Can you work these out from the model? Positions are in its coordinate system, mm. A direction names the side the tool comes from. Give positions to 0.01 mm unless a question says otherwise; leave off trailing zeros. Order: outer loops, then holes, each group sorted by start corner. A loop starts at its lowest first (then second) coordinate and runs counter-clockwise, first axis right, second up. Notation, with made-up numbers: M 6,52.25 L 46,52.25 A22 cw 46,61.25 Z; hole C 2.5,37 d10. An arc over 180 degrees is marked long. Answer as a JSON object with one key per item and string values.
```python
from build123d import *

# Parameters (mm, degrees)
SKETCH2_R           = 21
BOSS_EXTRUDE1_DEPTH = 3.5
SKETCH4_R           = 5.5
SKETCH4_R_2         = 1.143
SKETCH4_R_3         = 1.5875
CUT_EXTRUDE2_DEPTH  = 4.5
SKETCH5_R           = 2.9
CUT_EXTRUDE4_DEPTH  = 2
SKETCH6_W           = 2.148549125
SKETCH6_H           = 1
SKETCH8_R           = 3.6
SKETCH8_W           = 3.4
SKETCH8_H           = 3.4
BOSS_EXTRUDE3_DEPTH = 15
SKETCH7_R           = 6.25
BOSS_EXTRUDE4_DEPTH = 2.5


with BuildPart() as part:
    # Sketch2 → Boss-Extrude1 (new body)
    with BuildSketch(Plane(origin=(0, 0, 0), x_dir=(1, 0, 0), z_dir=(0, 1, 0))):
        Circle(SKETCH2_R)
    extrude(amount=BOSS_EXTRUDE1_DEPTH)

    # Sketch4 → Cut-Extrude2 (cut, through all)
    with BuildSketch(Plane(origin=(0, 3.5, 0), x_dir=(1, 0, 0), z_dir=(0, 1, 0))):
        Circle(SKETCH4_R)
        with Locations((7.445, 0)):
            Circle(SKETCH4_R_2)
        with Locations((10.54, 0)):
            Circle(SKETCH4_R_2)
        with Locations((13.46, 0)):
            Circle(SKETCH4_R_2)
        with Locations((16.51, 0)):
            Circle(SKETCH4_R_2)
        with Locations((10, 10)):
            Circle(SKETCH4_R_3)
        with Locations((0, -7.445)):
            Circle(SKETCH4_R_2)
        with Locations((0, -10.54)):
            Circle(SKETCH4_R_2)
        with Locations((0, -13.46)):
            Circle(SKETCH4_R_2)
        with Locations((0, -16.51)):
            Circle(SKETCH4_R_2)
        with Locations((10, -10)):
            Circle(SKETCH4_R_3)
        with Locations((-7.445, 0)):
            Circle(SKETCH4_R_2)
        with Locations((-10.54, 0)):
            Circle(SKETCH4_R_2)
        with Locations((-13.46, 0)):
            Circle(SKETCH4_R_2)
        with Locations((-16.51, 0)):
            Circle(SKETCH4_R_2)
        with Locations((-10, -10)):
            Circle(SKETCH4_R_3)
        with Locations((0, 7.445)):
            Circle(SKETCH4_R_2)
        with Locations((0, 10.54)):
            Circle(SKETCH4_R_2)
        with Locations((0, 13.46)):
            Circle(SKETCH4_R_2)
        with Locations((0, 16.51)):
            Circle(SKETCH4_R_2)
        with Locations((-10, 10)):
            Circle(SKETCH4_R_3)
    extrude(amount=-CUT_EXTRUDE2_DEPTH, mode=Mode.SUBTRACT)

    # Sketch5 → Cut-Extrude4 (cut)
    with BuildSketch(Plane(origin=(0, 3.5, 0), x_dir=(1, 0, 0), z_dir=(0, 1, 0))):
        with Locations((-10, 10)):
            Circle(SKETCH5_R)
        with Locations((-10, -10)):
            Circle(SKETCH5_R)
        with Locations((10, 10)):
            Circle(SKETCH5_R)
        with Locations((10, -10)):
            Circle(SKETCH5_R)
    extrude(amount=-CUT_EXTRUDE4_DEPTH, mode=Mode.SUBTRACT)

    # Sketch6 → Revolve1 (revolve)
    with BuildSketch(Plane.XY):
        with Locations((-21.425725437, 3)):
            Rectangle(SKETCH6_W, SKETCH6_H)
    revolve(axis=Axis((0, 0, 0), (0, 1, 0)))



with BuildPart() as body_2:
    # Sketch8 → Boss-Extrude3 (new body)
    with BuildSketch(Plane(origin=(0, 0, 0), x_dir=(1, 0, 0), z_dir=(0, 1, 0))):
        Circle(SKETCH8_R)
        Rectangle(SKETCH8_W, SKETCH8_H, mode=Mode.SUBTRACT)
    extrude(amount=BOSS_EXTRUDE3_DEPTH)


with BuildPart() as part_1:
    add(part.part)

    add(body_2.part)  # Boss-Extrude4 merges body 2
    # Sketch7 → Boss-Extrude4 (add)
    with BuildSketch(Plane(origin=(0, 3.5, 0), x_dir=(1, 0, 0), z_dir=(0, 1, 0))):
        Circle(SKETCH7_R)
    extrude(amount=-BOSS_EXTRUDE4_DEPTH)


solid = part_1.part
```
1) I need wall thicknesses on L1, parallel to X at y = 7.5, z = 0; L2, parallel to Y at x = -7.5, z = -19.5; L3, parallel to X at y = 0.55, z = 10. Which ranges of each line are inside material? Lowest first, please.
Results found:
{"L1": "x = -3.6 to -1.7, 1.7 to 3.6", "L2": "y = 0 to 3.5", "L3": "x = -18.47 to -11.59, -8.41 to -1.01, 1.01 to 8.41, 11.59 to 18.47"}
2) Thinking about a two-plate mould opening in Z: for faces 4 (the face through (3.434, 9.17, -1.081)), 5 (the face through (11.596, 1.774, 0.438)), which applies, pulls with the +Z half, pulls with the -Z half, needs draft (parallel to the pull), parting line crosses it, or undercut?
Results found:
{"face 4": "parting line crosses it", "face 5": "undercut"}
3) I want a section at C-C on x = 17. Write out the boundary of the cut face in (y, z).
Results found:
{"outline": "M 0,-12.33 L 2.5,-12.33 L 2.5,-14.74 L 3.5,-14.74 L 3.5,-1.03 L 0,-1.03 Z; M 0,1.03 L 3.5,1.03 L 3.5,14.74 L 2.5,14.74 L 2.5,12.33 L 0,12.33 Z"}
4) For faces 1 (the face through (11.25, 1.5, 11.25)), 2 (the face through (0, 0.5, 1.7)), 3 (the face through (-10.207, 0.76, 8.426)), which set-ups out of +Z, -Z, +X, -X, +Y, -Y let a thin tool reach every point of the face, with its end or its side?
Results found:
{"face 1": "+Y", "face 2": "-Y", "face 3": "+Y, -Y"}
5) I want a section at B-B on z = -10.54. Write out the boundary of the cut face in (x, y), and give its area (3 significant figures).
Results found:
{"outline": "M -19.88,2.5 L -18.16,2.5 L -18.16,0 L -11.49,0 L -11.49,1.5 L -12.85,1.5 L -12.85,3.5 L -19.88,3.5 Z; M -8.51,0 L -1.14,0 L -1.14,3.5 L -7.15,3.5 L -7.15,1.5 L -8.51,1.5 Z; M 1.14,0 L 8.51,0 L 8.51,1.5 L 7.15,1.5 L 7.15,3.5 L 1.14,3.5 Z; M 11.49,0 L 18.16,0 L 18.16,2.5 L 19.88,2.5 L 19.88,3.5 L 12.85,3.5 L 12.85,1.5 L 11.49,1.5 Z", "area": "90.8 mm²"}
6) I want a section at D-D on x = -10.54. Write out the boundary of the cut face in (y, z).
Results found:
{"outline": "M 0,-18.16 L 2.5,-18.16 L 2.5,-19.88 L 3.5,-19.88 L 3.5,-12.85 L 1.5,-12.85 L 1.5,-11.49 L 0,-11.49 Z; M 0,-8.51 L 1.5,-8.51 L 1.5,-7.15 L 3.5,-7.15 L 3.5,-1.14 L 0,-1.14 Z; M 0,1.14 L 3.5,1.14 L 3.5,7.15 L 1.5,7.15 L 1.5,8.51 L 0,8.51 Z; M 0,11.49 L 1.5,11.49 L 1.5,12.85 L 3.5,12.85 L 3.5,19.88 L 2.5,19.88 L 2.5,18.16 L 0,18.16 Z"}
7) I'm going to push flat-ended pins straight in: pin 1 Ø2 at (x, z) = (0, -7.445) entering from -Y; pin 2 Ø3.5 at (x, z) = (-10, 10) entering from +Y; pin 3 Ø6.5 at (x, z) = (11, 10.5) entering from +Y; pin 4 Ø1 at (x, y) = (0, 9) entering from +Z. Where does each tip first touch, or does it pass through?
Results found:
{"pin 1": "passes through", "pin 2": "stops at y = 1.5", "pin 3": "stops at y = 3.5", "pin 4": "stops at z = 3.6"}
8) I want a section at A-A on y = 7. Write out the boundary of the cut face in (x, z).
Results found:
{"outline": "C 0,0 d7.2; hole M -1.7,-1.7 L 1.7,-1.7 L 1.7,1.7 L -1.7,1.7 Z"}
